```python
from build123d import *

# Parameters (mm, degrees)
F1_DEPTH = 50.8
F2_W     = 50.8
F2_H     = 101.6
F3_DEPTH = 101.603284
F4_R     = 6.35
F5_DEPTH = 25.4
F6_R     = 6.35
F7_DEPTH = 12.7
F8_R     = 6.35
F9_DEPTH = 12.7


with BuildPart() as f1:
    # F0 (on Right) → F1 (new body, symmetric)
    with BuildSketch(Plane.YZ):
        Polygon((11.138843, 63.5), (-25.4, 63.5), (-25.4, -38.1), (-50.797716, -38.1), (-50.797716, -50.8), (76.202284, -50.8), (76.202284, -38.1), (63.502284, -38.1), align=None)
    extrude(amount=F1_DEPTH, both=True)

    # F2 (on face) → F3 (cut, through all)
    with BuildSketch(Plane.XZ.offset(25.4)):
        with Locations((0, 12.7)):
            Rectangle(F2_W, F2_H)
    extrude(amount=-F3_DEPTH, mode=Mode.SUBTRACT)

    # F4 (on Right) → F5 (join, symmetric)
    with BuildSketch(Plane.YZ):
        with Locations((-8.776936, 37.846457)):
            Circle(F4_R)
    extrude(amount=F5_DEPTH, both=True)

    # F6 (on face) → F7 (join)
    with BuildSketch(Plane.YZ.offset(-25.4)):
        with Locations((25.389081, -27.005039)):
            Circle(F6_R)
    extrude(amount=F7_DEPTH)

    # F8 (on face) → F9 (join)
    with BuildSketch(Plane(origin=(25.4, 0, 0), x_dir=(0, -1, 0), z_dir=(-1, 0, 0))):
        with Locations((-25.4, -27.040878)):
            Circle(F8_R)
    extrude(amount=F9_DEPTH)


solid = f1.part
```
Input: part model. Units: mm. Frame: model coordinates. A direction names the side the tool comes from. Give positions to 0.01 mm unless a question says otherwise; leave off trailing zeros. Loops run counter-clockwise (first coordinate to the right, second up) from the corner with the lowest first, then second, coordinate; pieces in that order, holes last.
1) Section query D-D on y = 36.5. Return the cut outline in (x, z), and give its area (3 significant figures).
A:
outline: (-50.8, -50.8) - (50.8, -50.8) - (50.8, 14.29) - (25.4, 14.29) - (25.4, -38.1) - (-25.4, -38.1) - (-25.4, 14.29) - (-50.8, 14.29) - close
area: 3,950 mm2
2) Section query C-C on x = -2. Return the cut outline in (y, z).
A:
outline: (-50.8, -50.8) - (76.2, -50.8) - (76.2, -38.1) - (-50.8, -38.1) - close; circle Ø12.7 at (-8.78, 37.85)
3) Section query B-B on x = -42.5. Return the cut outline in (y, z), and give its area (3 significant figures).
A:
outline: (-50.8, -50.8) - (76.2, -50.8) - (76.2, -38.1) - (63.5, -38.1) - (11.14, 63.5) - (-25.4, 63.5) - (-25.4, -38.1) - (-50.8, -38.1) - close
area: 7,990 mm2
4) Contact query for flat-ended pins moving along their axis: pin 1 (6 mm diameter, centred on x = -23, y = -31, fed in from +Z); pin 2 (12.5 mm diameter, centred on x = -44, z = 22.5, fed in from -Y). Output: stop coordinate, or through.
A:
pin 1: stops at z = -38.1
pin 2: stops at y = -25.4
5) Section query A-A on z = 1. Return the cut outline in (x, y), and give its area (3 significant figures).
A:
outline: (-50.8, -25.4) - (-25.4, -25.4) - (-25.4, 43.35) - (-50.8, 43.35) - close; (25.4, -25.4) - (50.8, -25.4) - (50.8, 43.35) - (25.4, 43.35) - close
area: 3,490 mm2
6) Mould query, pull axis Z, two halves, no side actions, for faces 1 (the flat face through (38, -7, 63.5)), 2 (the cylindrical face through (-19.139, 19.045, -26.726)), 3 (the flat face through (12.7, 25, -27)). Classes: released by +Z, released by -Z, zero draft, split by the parting line, or undercut.
A:
face 1: released by +Z
face 2: undercut
face 3: zero draft
7) Line query: L1, parallel to X at y = 46, z = -35.5; L2, parallel to Z at x = 18.5, y = 70; L3, parallel to Y at x = -29, z = -10.5. Output: solid intervals per line, ascending.
A:
L1: x = -50.8 to -25.4, 25.4 to 50.8
L2: z = -50.8 to -38.1
L3: y = -25.4 to 49.28
8) Reachability of faces 4 (the cylindrical face through (0.36, -2.72, 39.75)), 5 (the flat face through (-38, -25.4, 13)), 6 (the flat face through (-12.7, 25, -27)), 7 (the flat face through (-37.922, 37.687, 11.989)) from +Z, -Z, +X, -X, +Y, -Y: full face, straight path, thin tool, end or side. Return the list, or none.
A:
face 4: none
face 5: +Z, +X, -X, -Y
face 6: +Z, +Y, -Y
face 7: +Z, +X, -X, +Y
